Check sheet for the modelled part. Datum: model origin and axes. Units: mm. A direction names the side the tool comes from. Give positions to 0.01 mm unless a question says otherwise; leave off trailing zeros. Loops run counter-clockwise (first coordinate to the right, second up) from the corner with the lowest first, then second, coordinate; pieces in that order, holes last. Notation, with made-up numbers: M 49,-40 L 60,-40 A16 ccw 60,-34 Z; hole C 75.25,42 d2. An arc over 180 degrees is marked long. Put each result on its own line as item: value. Start each with the question number.
```python
from build123d import *

# Parameters (mm, degrees)
SKETCH1_R           = 91.44
BOSS_EXTRUDE1_DEPTH = 12.7
CUT_EXTRUDE1_DEPTH  = 12.7


with BuildPart() as part:
    # Sketch1 → Boss-Extrude1 (new body)
    with BuildSketch(Plane(origin=(0, 0, 0), x_dir=(0, 0, -1), z_dir=(1, 0, 0))):
        Circle(SKETCH1_R)
    extrude(amount=BOSS_EXTRUDE1_DEPTH)

    # Sketch2 → Cut-Extrude1 (cut)
    with BuildSketch(Plane(origin=(12.7, 0, 0), x_dir=(0, 0, -1), z_dir=(1, 0, 0))):
        with BuildLine():
            Line((7.62, 37.33022368), (7.62, 30.48))
            Line((7.62, 30.48), (-7.62, 30.48))
            Line((-7.62, 30.48), (-7.62, 37.33022368))
            ThreePointArc((-7.62, 37.33022368), (0, -38.1), (7.62, 37.33022368))
        make_face()
    extrude(amount=-CUT_EXTRUDE1_DEPTH, mode=Mode.SUBTRACT)


solid = part.part
```
Q1. Depth check by flat-ended pin: P1, Ø6, axis at x = 5, z = -17, coming from the +Y side; P2, Ø5.5, axis at x = 4, y = 35, coming from the -Z side; P3, Ø5.5, axis at x = 4, y = 34.5, coming from the +Z side; P4, Ø1, axis at y = -35.5, z = 4.5, coming from the -X side. Enter the tip coordinate at first touch or a pass-through.
Q2. Mould release check, pull along Y, two halves, no side actions. Record for faces 1 (the face through (0, -39, 1)), 2 (the face through (6, 34, 7.62)), 3 (the face through (6.261, 27.466, -87.217)): pulls with the +Y half, pulls with the -Y half, needs draft (parallel to the pull), parting line crosses it, or undercut.
Q3. Section check A-A, the plane y = 0. Record the cut outline in (x, z).
Q4. Access from +Z, -Z, +X, -X, +Y, -Y to the whole of each face (thin tool, end or side, straight path). Record for faces 4 (the face through (6, 34, -7.62)), 5 (the face through (12.7, -39, 1)).
Q5. Section check B-B, the plane z = 0. Record the cut outline in (x, y).
Q6. Thickness scan on line 1 along Y through (x, z) = (7.25, 0); line 2 along Z through (x, y) = (0.5, -1.5); line 3 along Z through (x, y) = (8.75, -34). Record the ranges inside material, lowest first. Write a range as [from, to].
Q7. Section check C-C, the plane x = 9. Record the cut outline in (y, z), then the cut area to 3 significant figures.
Q8. Section check D-D, the plane z = -78. Record the cut outline in (x, y).
Found:
1. P1: stops at y = 90.36
1. P2: stops at z = -85.56
1. P3: stops at z = 85.75
1. P4: passes through
2. face 1: needs draft
2. face 2: undercut
2. face 3: parting line crosses it
3. outline: M 0,-91.44 L 12.7,-91.44 L 12.7,-38.1 L 0,-38.1 Z; M 0,38.1 L 12.7,38.1 L 12.7,91.44 L 0,91.44 Z
4. face 4: +X, -X
4. face 5: +Z, -Z, +X, +Y, -Y
5. outline: M 0,-91.44 L 12.7,-91.44 L 12.7,-38.1 L 0,-38.1 Z; M 0,30.48 L 12.7,30.48 L 12.7,91.44 L 0,91.44 Z
6. line 1: y = [-91.44, -38.1], [30.48, 91.44]
6. line 2: z = [-91.43, -38.07], [38.07, 91.43]
6. line 3: z = [-84.88, -17.19], [17.19, 84.88]
7. outline: C 0,0 d182.88; hole M 30.48,-7.62 L 30.48,7.62 L 37.33,7.62 A38.1 ccw long 37.33,-7.62 Z
7. area: 21,800 mm^2
8. outline: M 0,-47.72 L 12.7,-47.72 L 12.7,47.72 L 0,47.72 Z
